Read the model definition and answer for the solid it produces. Units are mm, in the model's axes. Round coordinates to 2 decimals unless told otherwise and drop trailing zeros. Write each loop counter-clockwise with the first axis right and the second up, starting at its lowest first coordinate (ties: lowest second). Pieces come first, ordered by that corner, then holes. Notation, with made-up numbers: (-35, 12.25) -> (-6, 12.25) arc R10 cw to (-6, 27.25) -> close; hole circle Ø9 at (-31, 14). An arc over 180 degrees is marked (long way). Return JSON: item names as keys, results as strings. Group by question number.
(1) A cutting plane is placed at C-C on y = 21. Give the vertices of the cut face in (x, z), then the cut area to 3 significant figures.
(2) A cutting plane is placed at A-A on z = 1.55. Give the vertices of the cut face in (x, y).
(3) A cutting plane is placed at B-B on x = 89. Give the vertices of the cut face in (y, z).
(4) Straight lines are drawn through the part: line 1 (X direction, y = 5.5, z = 3.15); line 2 (Y direction, x = 68.5, z = 1.7); line 3 (Y direction, x = 51, z = 4.6). For each, find the intervals that lie inside material, in ascending order.
(5) Given pin 1 (1.5 mm diameter, centred on y = -4, z = 3.5, fed in from +X); pin 2 (1.5 mm diameter, centred on x = 91.5, y = 6, fed in from -Z); pin 3 (1.5 mm diameter, centred on x = 62, z = 3, fed in from -Y), each flat-ended and moving along its own axis, determine where each tip first touches the part or whether it passes through.
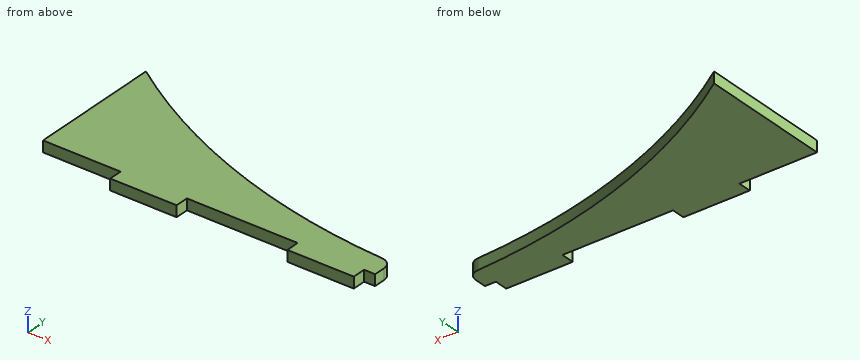
```python
from build123d import *

# Parameters (mm, degrees)
EXTRUDE_1_DEPTH = 5
FILLET_1_R      = 5


with BuildPart() as part:
    # 草图1 → 凸台-拉伸1 (new body)
    with BuildSketch(Plane.XY):
        with BuildLine():
            Line((125, 0), (125, -6))
            Line((125, -6), (95, -6))
            Line((95, -6), (95, 0))
            Line((95, 0), (45, 0))
            Line((45, 0), (45, -6))
            Line((45, -6), (15, -6))
            Line((15, -6), (15, 0))
            Line((15, 0), (0, 0))
            Line((0, 0), (-20, 0))
            Line((-20, 0), (-20, 60))
            ThreePointArc((-20, 60), (51.397381618, 24.192144853), (130, 10))
            Line((130, 10), (130, 0))
            Line((130, 0), (125, 0))
        make_face()
    extrude(amount=EXTRUDE_1_DEPTH)

    # 圆角1
    fillet_1_edges = [part.edges().sort_by_distance(p)[0] for p in [
        (130, 10, 2.5),
    ]]
    fillet(fillet_1_edges, radius=FILLET_1_R)


solid = part.part
```
Checks:
{
 "1": {"outline": "(-20, 0) -> (61.62, 0) -> (61.62, 5) -> (-20, 5) -> close", "area": "408 mm^2"},
 "2": {"outline": "(-20, 0) -> (15, 0) -> (15, -6) -> (45, -6) -> (45, 0) -> (95, 0) -> (95, -6) -> (125, -6) -> (125, 0) -> (130, 0) -> (130, 5.22) arc R5 ccw to (125.26, 10.21) arc R280 cw to (-20, 60) -> close"},
 "3": {"outline": "(0, 0) -> (14.5, 0) -> (14.5, 5) -> (0, 5) -> close"},
 "4": {"line 1": "x = -20 to 129.99", "line 2": "y = 0 to 19.09", "line 3": "y = 0 to 24.32"},
 "5": {"pin 1": "stops at x = 125", "pin 2": "stops at z = 0", "pin 3": "stops at y = 0"}
}
